Source: CAD feature listing. Evaluate the final solid. Frame: model axes, mm. A direction names the side the tool comes from. Give positions to 0.01 mm unless a question says otherwise; leave off trailing zeros. Loops run counter-clockwise (first coordinate to the right, second up) from the corner with the lowest first, then second, coordinate; pieces in that order, holes last. Notation, with made-up numbers: (7.5, 12) - (49.5, 12) arc R26 ccw to (49.5, 26) - close; hole circle Ø7 at (57.5, 15). An arc over 180 degrees is marked (long way). Put each result on its own line as item: value.
Autodesk Inventor part; units mm, degrees
ref_plane "YZ Plane" through (0, 0, 0) normal (1, 0, 0) x (0, 1, 0)
ref_plane "XZ Plane" through (0, 0, 0) normal (0, 1, 0) x (-1, 0, 0)
ref_plane "XY Plane" through (0, 0, 0) normal (0, 0, 1) x (1, 0, 0)
sketch "Sketch1" plane through (0, 0, 0) normal (1, 0, 0) x (0, 1, 0)
  point P0 (0, 0)
sketch "Sketch2" plane through (0, 0, 0) normal (1, 0, 0) x (0, 1, 0)
  line L0 (-54.61, 7.9375) -> (54.61, 7.9375)
  line L1 (54.61, 7.9375) -> (54.61, -7.9375)
  line L2 (54.61, -7.9375) -> (-54.61, -7.9375)
  line L3 (-54.61, -7.9375) -> (-54.61, 7.9375)
  line L4 (-54.61, 7.9375) -> (54.61, -7.9375) construction
  line L5 (54.61, 7.9375) -> (-54.61, -7.9375) construction
  point P0 (0, 0)
  dimension "d0" = 15.875
  dimension "d1" = 109.22
extrude "Extrusion1" add sketch "Sketch2" along normal blind 3.175
sketch "Sketch3" plane through (3.175, -54.61, 7.9375) normal (0, 0, 1) x (1, 0, 0)
  line L0 (0, 109.22) -> (0, 0)
  line L1 (0, 0) -> (15.875, 0)
  line L2 (15.875, 0) -> (15.875, 109.22)
  line L3 (15.875, 109.22) -> (0, 109.22)
edge flange "Flange1" height 19.05 angle 90 thickness 3.175 bend radius 1.27 thickness toward (0, 0, 1) relief tear relief width 3.175 relief depth 1.5875 edges at (3.175, 0, 7.9375) wall of the first edge with corners at (3.175, 54.61, 7.9375) (3.175, -54.61, 7.9375) (19.05, -54.61, 7.9375) (19.05, 54.61, 7.9375)
bend "Bend1"
corner "Corner1"
sketch "Sketch4" plane through (3.175, 0, 0) normal (1, 0, 0) x (0, 0, -1)
  line L0 (1.9431, 29.21) -> (1.9431, -29.21) construction
  line L1 (7.9375, -54.61) -> (7.9375, 54.61) construction
  line L2 (7.9375, 54.61) -> (-6.6675, 54.61)
  line L3 (-6.6675, -54.61) -> (7.9375, -54.61)
  point P0 (0, 0)
  dimension "d14" = 5.9944
  dimension "d15" = 25.4
  dimension "d16" = 25.4
hole "Hole1" at (3.175, 29.21, -1.9431) at (3.175, -29.21, -1.9431) direction (-1, 0, 0) diameter 6 end through all
sketch "Sketch5" plane through (19.05, -54.61, 7.9375) normal (0, 0, -1) x (-1, 0, 0)
  line L0 (5.9944, 12.7) -> (5.9944, 96.52) construction
  line L1 (0, 109.22) -> (0, 0) construction
  line L2 (0, 109.22) -> (14.605, 109.22) construction
  line L3 (0, 0) -> (14.605, 0) construction
  point P0 (19.05, 54.61)
  dimension "d24" = 5.9944
  dimension "d25" = 12.7
  dimension "d26" = 12.7
hole "Hole2" at (13.0556, 41.91, 7.9375) at (13.0556, -41.91, 7.9375) direction (0, 0, 1) diameter 6 end through all
sketch "Sketch6" plane through (3.175, 0, 0) normal (1, 0, 0) x (0, 0, -1)
  circle A0 centre (1.9431, 29.21) radius 3
  point P0 (0, 0)
  point P1 (4.9431, 29.21)
equation "\"d22\" = Thickness"
equation "\"d32\" = Thickness"
equation "\"d4\" = BendReliefWidth"
equation "\"d5\" = BendReliefDepth"
equation "\"d6\" = MinimumRemnant"
equation "\"d7\" = BendRadius"
equation "\"d11\" = CornerReliefSize"
equation "\"d12\" = GapSize"
equation "\"d13\" = JacobiRadiusSize"
equation "\"BendRadius\" = Thickness"
equation "\"BendReliefWidth\" = Thickness"
equation "\"BendReliefDepth\" = 0.5 * Thickness"
equation "\"CornerReliefSize\" = 4 * Thickness"
equation "\"MinimumRemnant\" = 2 * Thickness"
equation "\"TransitionRadius\" = BendRadius"
equation "\"JacobiRadiusSize\" = BendRadius"
equation "\"GapSize\" = Thickness"
properties part number "PCB_brackets" material "Aluminum 6061"
1) Material intervals for line 1 along X through (y, z) = (28.5, 2.25) (3 decimals); line 2 along Z through (x, y) = (0.9, -29.21); line 3 along Z through (x, y) = (2.45, 29.21), sorted ascending. Write a range as [from, to].
Check result:
line 1: [0, 3.175]
line 2: [-7.94, -4.94], [1.06, 9.35]
line 3: [-7.94, -4.94], [1.06, 10.64]
2) Access query for faces 1 (the flat face through (12, -1, 7.938)), 2 (the flat face through (19.05, -1, 10)). Directions: +Z, -Z, +X, -X, +Y, -Y. A direction counts if a zero-diameter tool reaches every point of the face in a straight line with its end or side. Return the directions, or none.
Check result:
face 1: -Z, +X, +Y, -Y
face 2: +Z, -Z, +X, +Y, -Y
3) Section query B-B, the plane z = -4. Output: boundary loops of the cut face in (x, y) (3 decimals).
Check result:
outline: (0, -54.61) - (3.175, -54.61) - (3.175, -31.394) - (0, -31.394) - close; (0, -27.026) - (3.175, -27.026) - (3.175, 27.026) - (0, 27.026) - close; (0, 31.394) - (3.175, 31.394) - (3.175, 54.61) - (0, 54.61) - close
4) Section query D-D, the plane z = 2.5. Output: boundary loops of the cut face in (x, y) (3 decimals), plus the area to 3 significant figures.
Check result:
outline: (0, -54.61) - (3.175, -54.61) - (3.175, 54.61) - (0, 54.61) - close
area: 347 mm²
5) Pin query (flat end, axial travel): P1, Ø1.5, axis at x = 4.5, y = -33.5, coming from the -Z side; P2, Ø10, axis at x = 15, y = -0.5, coming from the -Z side. Return the tip coordinate at first contact, or that it passes through.
Check result:
P1: z = 7.73
P2: z = 7.94
6) Section query C-C, the plane x = 17. Output: boundary loops of the cut face in (y, z).
Check result:
outline: (-54.61, 7.94) - (54.61, 7.94) - (54.61, 11.11) - (-54.61, 11.11) - close
7) Mould query, pull axis Y, two halves, no side actions, for faces 3 (the cylindrical face through (1.337, -0.765, 9.845)), 4 (the flat face through (7, -54.61, 9)), 5 (the cylindrical face through (1.57, 32.14, -1.29)). Classes: pulls with the +Y half, pulls with the -Y half, needs draft (parallel to the pull), parting line crosses it, or undercut.
Check result:
face 3: needs draft
face 4: pulls with the -Y half
face 5: undercut
